Geometry check sheet. Reference: the model listing, model coordinates, mm. A direction names the side the tool comes from. Give positions to 0.01 mm unless a question says otherwise; leave off trailing zeros. Write each loop counter-clockwise with the first axis right and the second up, starting at its lowest first coordinate (ties: lowest second). Pieces come first, ordered by that corner, then holes. Notation, with made-up numbers: (42, -30.5) -> (80, -30.5) arc R11 ccw to (80, -20.5) -> close; hole circle Ø3 at (24, 30). An arc over 180 degrees is marked (long way). Write item = value, one per line. Start each with the question number.
1. Cross-section at D-D, the plane y = 15.25. Record the cut outline in (x, z).
2. Cross-section at C-C, the plane x = 47.5. Record the cut outline in (y, z).
3. Set-up check for faces 1 (the flat face through (8, 10, -4)), 2 (the flat face through (58, 10, 0)), 3 (the flat face through (10, -5, 4)), 4 (the flat face through (46, 10, 7.8)), 5 (the cylindrical face through (31, -5, 6)): record each of +Z, -Z, +X, -X, +Y, -Y from which the full face is reachable in a straight line by a thin tool's end or side.
4. Thickness scan on line 1 along Y through (x, z) = (29, 4); line 2 along Z through (x, y) = (31.5, 7.25); line 3 along Z through (x, y) = (9, 1). Record the ranges inside material, lowest first.
5. Cross-section at B-B, the plane x = 4.5. Record the cut outline in (y, z).
6. Mould release check, pull along Z, two halves, no side actions. Record for faces 6 (the flat face through (0, 9, 4)), 7 (the cylindrical face through (4.93, -2.97, 1.79)), 8 (the flat face through (4, 10, 0)): pulls with the +Z half, pulls with the -Z half, needs draft (parallel to the pull), parting line crosses it, or undercut.
7. Depth check by flat-ended pin: P1, Ø6.5, axis at x = 2, y = 10.5, coming from the -Z side; P2, Ø2, axis at x = 8.5, y = 5.5, coming from the -Z side; P3, Ø4, axis at x = 54.5, z = -3, coming from the -Y side. Enter the tip coordinate at first touch or a pass-through.
8. Cross-section at A-A, the plane x = 32.5. Record the cut outline in (y, z), plus the area to 3 significant figures.
Autodesk Inventor part; units mm, degrees
ref_plane "YZ Plane" through (0, 0, 0) normal (1, 0, 0) x (0, 1, 0)
ref_plane "XZ Plane" through (0, 0, 0) normal (0, 1, 0) x (-1, 0, 0)
ref_plane "XY Plane" through (0, 0, 0) normal (0, 0, 1) x (1, 0, 0)
sketch "スケッチ1" plane through (0, 0, 0) normal (0, 0, 1) x (1, 0, 0)
  line L0 (0, 0) -> (62, 0)
  line L1 (62, 0) -> (62, 20)
  line L2 (62, 20) -> (0, 20)
  line L3 (0, 20) -> (0, 0)
  dimension "d0" = 62
  dimension "d1" = 20
extrude "押し出し1" add sketch "スケッチ1" along normal blind 8
sketch "スケッチ2" plane through (0, 0, 0) normal (-1, 0, 0) x (0, 0, 1)
  line L0 (0, 0) -> (8, 0)
  line L1 (4, 0) -> (4, -1)
  line L2 (4, -1) -> (4, -5) construction
  circle A0 centre (4, -5) radius 4
  line L3 (8, 0) -> (8, -5)
  circle A1 centre (4, -5) radius 3
  dimension "d4" = 1
  dimension "d5" = 4
  dimension "d6" = 6
extrude "押し出し2" add sketch "スケッチ2" against normal blind 20
sketch "スケッチ3" plane through (20, 0, 0) normal (1, 0, 0) x (0, 0, -1)
  arc A0 (-8, -5) -> (-4, -1) centre (-4, -5) ccw construction
  line L0 (0, 0) -> (-4, 0) construction
  line L1 (-4, 0) -> (-4, -5) construction
  line L2 (-4, -5) -> (0, -5) construction
  line L3 (0, -5) -> (0, 0) construction
  circle A1 centre (-4, -5) radius 3
extrude "押し出し3" add sketch "スケッチ3" along normal blind 2 and the other way blind 10
sketch "スケッチ4" plane through (22, -5, 4) normal (1, 0, 0) x (0, 0, -1)
  circle A0 centre (0, 0) radius 2
  circle A1 centre (0, 0) radius 1.5
  point P0 (4, 5)
  dimension "d13" = 4
  dimension "d14" = 3
extrude "押し出し4" add sketch "スケッチ4" along normal blind 18
sketch "スケッチ5" plane through (0, 0, 0) normal (0, 0, -1) x (-1, 0, 0)
  line L0 (0, 0) -> (-62, 0) construction
  line L1 (0, 0) -> (-8, 0) construction
  line L2 (-62, 0) -> (-54, 0) construction
  line L3 (-62, 20) -> (0, 20)
  line L4 (-8, 0) -> (-54, 0)
  line L5 (-54, 0) -> (-54, 20)
  line L6 (-54, 20) -> (-8, 20)
  line L7 (-8, 20) -> (-8, 0)
  dimension "d17" = 8
  dimension "d18" = 8
extrude "押し出し5" add sketch "スケッチ5" along normal blind 8
chamfer "面取り1" distance 3 distance2 8 1 edges at (31, 20, -8) measured on face at (23.3333, 6.6667, -8)
sketch "スケッチ6" plane through (0, 0, -8) normal (0, 0, -1) x (-1, 0, 0)
  line L0 (-54, 17) -> (-8, 17) construction
  line L1 (-8, 17) -> (-9.5, 17) construction
  line L2 (-9.5, 17) -> (-9.5, 16) construction
  line L3 (-9.5, 16) -> (-8, 16) construction
  line L4 (-8, 16) -> (-8, 17) construction
  line L5 (-9.5, 16) -> (-19, 16)
  line L6 (-19, 16) -> (-19, 10)
  line L7 (-19, 10) -> (-9.5, 10)
  line L8 (-9.5, 10) -> (-9.5, 16)
  point P0 (0, 0)
  dimension "d26" = 9.5
  dimension "d27" = 6
  dimension "d28" = 1.5
  dimension "d29" = 1
extrude "押し出し6" add sketch "スケッチ6" along normal blind 1
sketch "スケッチ7" plane through (0, 0, 8) normal (0, 0, 1) x (1, 0, 0)
  line L0 (0, 0) -> (0, 9) construction
  line L1 (0, 20) -> (0, 0) construction
  line L2 (0, 9) -> (25, 9)
  line L3 (25, 9) -> (25, 11)
  line L4 (25, 11) -> (0, 11)
  line L5 (0, 11) -> (0, 9)
  line L6 (20, 0) -> (62, 0) construction
  line L7 (62, 0) -> (60.5, 0) construction
  line L8 (60.5, 0) -> (60.5, 3) construction
  line L9 (60.5, 3) -> (62, 3) construction
  line L10 (62, 3) -> (62, 0) construction
  line L11 (60.5, 3) -> (31, 3)
  line L12 (31, 3) -> (31, 17)
  line L13 (31, 17) -> (60.5, 17)
  line L14 (60.5, 17) -> (60.5, 3)
  dimension "d32" = 9
  dimension "d33" = 25
  dimension "d34" = 2
  dimension "d37" = 1.5
  dimension "d38" = 3
  dimension "d39" = 29.5
  dimension "d40" = 14
extrude "押し出し8" cut sketch "スケッチ7" against normal blind 0.2
sketch "スケッチ9" plane through (0, 0, 7.8) normal (0, 0, 1) x (1, 0, 0)
  line L0 (31, 3) -> (31, 17) construction
  line L1 (31, 10) -> (40, 10) construction
  circle A0 centre (40, 10) radius 3
  line L2 (60.5, 17) -> (60.5, 3) construction
  line L3 (60.5, 10) -> (53, 10) construction
  line L4 (52.25, 9.5) -> (53.75, 9.5)
  line L5 (53.75, 9.5) -> (53.75, 10.5)
  line L6 (53.75, 10.5) -> (52.25, 10.5)
  line L7 (52.25, 10.5) -> (52.25, 9.5)
  line L8 (52.25, 9.5) -> (53.75, 10.5) construction
  line L9 (53.75, 9.5) -> (52.25, 10.5) construction
  point P0 (0, 0)
  dimension "d43" = 9
  dimension "d44" = 6
  dimension "d45" = 7.5
  dimension "d46" = 1.5
  dimension "d47" = 1
extrude "押し出し9" cut sketch "スケッチ9" against normal blind 0.3
thread "ねじ1"
properties part number "UCAM-DLI500TNBK"
Answers:
q1.outline = (0, 0) -> (8, 0) -> (8, -8) -> (9.5, -8) -> (9.5, -9) -> (19, -9) -> (19, -8) -> (54, -8) -> (54, 0) -> (62, 0) -> (62, 8) -> (60.5, 8) -> (60.5, 7.8) -> (31, 7.8) -> (31, 8) -> (0, 8) -> close
q2.outline = (0, -8) -> (17, -8) -> (20, 0) -> (20, 8) -> (17, 8) -> (17, 7.8) -> (3, 7.8) -> (3, 8) -> (0, 8) -> close
q3.face_1 = -Z, -X, +Y, -Y
q3.face_2 = -Z, +X, +Y, -Y
q3.face_3 = -X
q3.face_4 = +Z
q3.face_5 = +X
q4.line_1 = -7 to -6.5, -3.5 to -3, 0 to 20
q4.line_2 = -8 to 7.8
q4.line_3 = -8 to 8
q5.outline = (-5, 8) arc R4 ccw (long way) to (-1, 4) -> (0, 4) -> (0, 0) -> (20, 0) -> (20, 8) -> (11, 8) -> (11, 7.8) -> (9, 7.8) -> (9, 8) -> close; hole circle Ø6 at (-5, 4)
q6.face_6 = needs draft
q6.face_7 = undercut
q6.face_8 = pulls with the -Z half
q7.P1 = 0
q7.P2 = -8
q7.P3 = 0
q8.outline = circle Ø4 at (-5, 4); (0, -8) -> (17, -8) -> (20, 0) -> (20, 8) -> (17, 8) -> (17, 7.8) -> (3, 7.8) -> (3, 8) -> (0, 8) -> close; hole circle Ø3 at (-5, 4)
q8.area = 311 mm^2
